Here's how the part is built. I have some questions about the finished solid (model axes, mm). A direction names the side the tool comes from. Coordinates: 2 decimals unless noted, no trailing zeros. Write each loop counter-clockwise with the first axis right and the second up, starting at its lowest first coordinate (ties: lowest second). Pieces come first, ordered by that corner, then holes.
Item 1: I'm going to push flat-ended pins straight in: pin 1 Ø1.6 at (x, y) = (33, 1) entering from -Z; pin 2 Ø4 at (x, z) = (15.5, -11.5) entering from +Y; pin 3 Ø5 at (x, z) = (29, -11.5) entering from -Y; pin 4 Ø2 at (x, y) = (31, 1.5) entering from +Z. Where does each tip first touch, or does it pass through?
Item 2: If we section it at D-D (z = -8.5): Please give me the cut outline in (x, y).
Item 3: If we section it at B-B (z = -5): Please give me the cut outline in (x, y), then the cut area to 3 significant figures.
Item 4: If I drill on line 1 (X direction, y = 1.05, z = -5); line 2 (Y direction, x = 0, z = -0.75); line 3 (Z direction, x = 35.5, y = 1.1), over which ranges is the centre line in solid material (lowest first)?
Item 5: We'd pull the mould along X, two halves only. Please class faces 1 (the face through (38, 1, -5)), 2 (the face through (15, -3, -12)), 3 (the face through (29, 1, -5)): +X half, -X half, draft (parallel to the pull), parting line (faces both ways), or undercut.
Item 6: If we section it at A-A (x = 4): Please give me the cut outline in (y, z), then the cut area to 3 significant figures.
Item 7: For faces 4 (the face through (27.415, -0.465, -6.302)), 5 (the face through (32, 1, 0)), 6 (the face through (32, 1, -10)), which set-ups out of +Z, -Z, +X, -X, +Y, -Y let a thin tool reach every point of the face, with its end or its side?
Item 8: If we section it at C-C (y = 0.8): Please give me the cut outline in (x, z), then the cut area to 3 significant figures.
from build123d import *

# Parameters (mm, degrees)
SKETCH1_W           = 35
SKETCH1_H           = 10
BOSS_EXTRUDE1_DEPTH = 2
SKETCH2_R           = 10
BOSS_EXTRUDE2_DEPTH = 5
SKETCH3_R           = 7
CUT_EXTRUDE1_DEPTH  = 2000
SKETCH4_R           = 2
CUT_EXTRUDE2_DEPTH  = 20
SKETCH5_W           = 10
SKETCH5_H           = 2
BOSS_EXTRUDE3_DEPTH = 3
SKETCH6_W           = 10
SKETCH6_H           = 2
BOSS_EXTRUDE4_DEPTH = 3


with BuildPart() as part:
    # Sketch1 → Boss-Extrude1 (new body)
    with BuildSketch(Plane(origin=(0, 0, 0), x_dir=(1, 0, 0), z_dir=(0, 1, 0))):
        with Locations((17.5, 5)):
            Rectangle(SKETCH1_W, SKETCH1_H)
    extrude(amount=BOSS_EXTRUDE1_DEPTH)

    # Sketch2 → Boss-Extrude2 (add)
    with BuildSketch(Plane(origin=(0, 2, 0), x_dir=(1, 0, 0), z_dir=(0, 1, 0))):
        with Locations(Location((17.5, 5, 0), (0, 0, 270))):
            Circle(SKETCH2_R)
    extrude(amount=-BOSS_EXTRUDE2_DEPTH)

    # Sketch3 → Cut-Extrude1 (cut)
    with BuildSketch(Plane(origin=(0, 2, 0), x_dir=(1, 0, 0), z_dir=(0, 1, 0))):
        with Locations(Location((17.5, 5, 0), (0, 0, 270))):
            Circle(SKETCH3_R)
    extrude(amount=-CUT_EXTRUDE1_DEPTH, mode=Mode.SUBTRACT)

    # Sketch4 → Cut-Extrude2 (cut)
    with BuildSketch(Plane.XZ):
        with Locations(Location((4, -5, 0), (0, 0, 270))):
            Circle(SKETCH4_R)
        with Locations(Location((31, -5, 0), (0, 0, 270))):
            Circle(SKETCH4_R)
    extrude(amount=-CUT_EXTRUDE2_DEPTH, mode=Mode.SUBTRACT)

    # Sketch5 → Boss-Extrude3 (add)
    with BuildSketch(Plane.ZY):
        with Locations((-5, 1)):
            Rectangle(SKETCH5_W, SKETCH5_H)
    extrude(amount=BOSS_EXTRUDE3_DEPTH)

    # Sketch6 → Boss-Extrude4 (add)
    with BuildSketch(Plane(origin=(35, 0, 0), x_dir=(0, 0, -1), z_dir=(1, 0, 0))):
        with Locations((5, 1)):
            Rectangle(SKETCH6_W, SKETCH6_H)
    extrude(amount=BOSS_EXTRUDE4_DEPTH)


solid = part.part
Answer list:
1. pin 1: stops at z = -10
1. pin 2: stops at y = 2
1. pin 3: stops at y = 0
1. pin 4: stops at z = 0
2. outline: (-3, 0) - (8.13, 0) - (8.13, -3) - (11.44, -3) - (11.44, 2) - (-3, 2) - close; (23.56, -3) - (26.87, -3) - (26.87, 0) - (38, 0) - (38, 2) - (23.56, 2) - close
3. outline: (-3, 0) - (2, 0) - (2, 2) - (-3, 2) - close; (6, 0) - (7.5, 0) - (7.5, -3) - (10.5, -3) - (10.5, 2) - (6, 2) - close; (24.5, -3) - (27.5, -3) - (27.5, 0) - (29, 0) - (29, 2) - (24.5, 2) - close; (33, 0) - (38, 0) - (38, 2) - (33, 2) - close
3. area: 56.0 mm2
4. line 1: x = -3 to 2, 6 to 10.5, 24.5 to 29, 33 to 38
4. line 2: y = 0 to 2
4. line 3: z = -10 to 0
5. face 1: +X half
5. face 2: draft
5. face 3: undercut
6. outline: (0, -10) - (2, -10) - (2, -7) - (0, -7) - close; (0, -3) - (2, -3) - (2, 0) - (0, 0) - close
6. area: 12.0 mm2
7. face 4: -Y
7. face 5: +Z, +X, +Y, -Y
7. face 6: -Z, +X, +Y, -Y
8. outline: (-3, -10) - (8.84, -10) arc R10 ccw to (26.16, -10) - (38, -10) - (38, 0) - (26.16, 0) arc R10 ccw to (8.84, 0) - (-3, 0) - close; hole circle Ø4 at (4, -5); hole circle Ø14 at (17.5, -5); hole circle Ø4 at (31, -5)
8. area: 354 mm2
